Input: part model. Units: mm. Frame: model coordinates. A direction names the side the tool comes from. Give positions to 0.01 mm unless a question says otherwise; leave off trailing zeros. Write each loop counter-clockwise with the first axis right and the second up, starting at its lowest first coordinate (ties: lowest second). Pieces come first, ordered by that corner, then holes. Notation, with made-up numbers: (9, 34) - (40, 34) arc R34 cw to (40, 64) - close; hole circle Ø5 at (-37, -32.5). An arc over 180 degrees is marked (long way). Answer as a JSON object with one key per item and string values. Group by question number.
from build123d import *

# Parameters (mm, degrees)
SKETCH1_R                  = 2.430870735
SKETCH1_R_2                = 2.36295848
BASE_FLANGE1_DEPTH         = 1.0922
SKETCHED_START             = 12.060869776
SKETCHED_BEND3_OUTLINE_W   = 11.2522
SKETCHED_BEND3_OUTLINE_H   = 1.0922
SKETCHED_BEND3_DEPTH       = 16.450630224
SKETCHED_START_2           = 10.968669776
SKETCHED_BEND3_2_OUTLINE_R = 2.36295848
SKETCHED_BEND3_2_DEPTH     = 0.899042144
SKETCHED_START_3           = 10.232069776
SKETCHED_BEND3_3_OUTLINE_R = 2.36295848
SKETCHED_BEND3_3_DEPTH     = 1.8288
SKETCHED_START_4           = -5.6261
SKETCHED_BEND3_4_DEPTH     = 11.2522


with BuildPart() as part:
    # Base-Flange1: sheet metal written as solids
    # Sketch1 → Base-Flange1 (new body)
    with BuildSketch(Plane.XY):
        Polygon((-5.6261, 28.5115), (5.6261, 28.5115), (5.6261, 16.8275), (3.1242, 15.8115), (3.1242, 6.1595), (5.6261, 5.1435), (5.6261, -6.5405), (-5.6261, -6.5405), (-5.6261, 5.1435), (-3.1242, 6.1595), (-3.1242, 15.8115), (-5.6261, 16.8275), align=None)
        Circle(SKETCH1_R, mode=Mode.SUBTRACT)
        with Locations((0, 21.971)):
            Circle(SKETCH1_R_2, mode=Mode.SUBTRACT)
    extrude(amount=-BASE_FLANGE1_DEPTH)

    # Sketched Bend3: read off the stored shape, not the designer's step
    # Sketched Bend3 outline → Sketched Bend3 (cut)
    with BuildSketch(Plane(origin=(0, 0, 0), x_dir=(1, 0, 0), z_dir=(0, 1, 0)).offset(SKETCHED_START)):
        with Locations((0, 0.5461)):
            Rectangle(SKETCHED_BEND3_OUTLINE_W, SKETCHED_BEND3_OUTLINE_H)
    extrude(amount=SKETCHED_BEND3_DEPTH, mode=Mode.SUBTRACT)

    # Sketched Bend3 2 outline → Sketched Bend3 2 (add)
    with BuildSketch(Plane(origin=(0, 0, 0), x_dir=(1, 0, 0), z_dir=(0, 1, 0)).offset(SKETCHED_START_2)):
        Polygon((5.6261, 18.093369776), (-5.6261, 18.093369776), (-5.6261, 6.409369776), (-3.1242, 5.393369776), (-3.1242, 1.0922), (3.1242, 1.0922), (3.1242, 5.393369776), (5.6261, 6.409369776), align=None)
        with Locations((0, 11.552869776)):
            Circle(SKETCHED_BEND3_2_OUTLINE_R, mode=Mode.SUBTRACT)
    extrude(amount=SKETCHED_BEND3_2_DEPTH)

    # Sketched Bend3 3 outline → Sketched Bend3 3 (add)
    with BuildSketch(Plane(origin=(0, 0, 0), x_dir=(1, 0, 0), z_dir=(0, 1, 0)).offset(SKETCHED_START_3)):
        Polygon((5.6261, 18.093369776), (-5.6261, 18.093369776), (-5.6261, 6.409369776), (-3.1242, 5.393369776), (-3.1242, 1.0922), (3.1242, 1.0922), (3.1242, 5.393369776), (5.6261, 6.409369776), align=None)
        with Locations((0, 11.552869776)):
            Circle(SKETCHED_BEND3_3_OUTLINE_R, mode=Mode.SUBTRACT)
    extrude(amount=SKETCHED_BEND3_3_DEPTH)

    # Sketched Bend3 4 outline → Sketched Bend3 4 (cut)
    with BuildSketch(Plane.YZ.offset(SKETCHED_START_4)):
        with BuildLine():
            ThreePointArc((10.232069776, 0), (11.525226657, -0.535643119), (12.060869776, -1.8288))
            Line((12.060869776, -1.8288), (12.060869776, 0))
            Line((12.060869776, 0), (10.232069776, 0))
        make_face()
        with BuildLine():
            Line((10.968669776, -18.093369776), (10.968669776, -1.8288))
            ThreePointArc((10.968669776, -1.8288), (10.752924631, -1.307945145), (10.232069776, -1.0922))
            Line((10.232069776, -1.0922), (10.232069776, -18.093369776))
            Line((10.232069776, -18.093369776), (10.968669776, -18.093369776))
        make_face()
    extrude(amount=SKETCHED_BEND3_4_DEPTH, mode=Mode.SUBTRACT)


solid = part.part
1) Cut plane A-A on x = 0. Return the cut outline in (y, z), and give its area (3 significant figures).
2) Cut plane C-C on x = 1.75. Return the cut outline in (y, z).
3) Cut plane D-D on z = -8.5. Return the cut outline in (x, y).
4) Reachability of faces 5 (the face through (3.124, 9.7, -0.9)), 6 (the face through (2.32, 0.73, -0.54)), 7 (the face through (0, 10.969, -8)), 8 (the face through (-3.124, 9.7, -0.9)) from +Z, -Z, +X, -X, +Y, -Y: full face, straight path, thin tool, end or side. Return the list, or none.
5) Pin query (flat end, axial travel): P1, Ø4.5, axis at y = 10, z = -2, coming from the -X side; P2, Ø3.5, axis at x = -1, z = -12.5, coming from the -Y side; P3, Ø1.6, axis at y = 10.5, z = -2, coming from the +X side. Return the tip coordinate at first contact, or that it passes through.
6) Line query: line 1 along Y through (x, z) = (-4.5, -12.5); line 2 along Y through (x, z) = (0, -0.75); line 3 along Z through (x, y) = (0, 11.8). Output: solid intervals per line, ascending. Write a range as from..to.
7) Cut plane B-B on y = 0. Return the cut outline in (x, z), and give its area (3 significant figures).
8) Mould query, pull axis X, two halves, no side actions, for faces 1 (the face through (0, 12.061, -8)), 2 (the face through (1.09, 11.507, -9.457)), 3 (the face through (-5.626, -0.8, -0.5)), 4 (the face through (5.626, 11.5, -12.2)). Classes: +X half, -X half, draft (parallel to the pull), parting line (faces both ways), or undercut.
Filled in:
{
 "1": {"outline": "(-6.54, -1.09) - (-2.43, -1.09) - (-2.43, 0) - (-6.54, 0) - close; (2.43, -1.09) - (10.23, -1.09) arc R0.74 cw to (10.97, -1.83) - (10.97, -9.19) - (12.06, -9.19) - (12.06, -1.83) arc R1.83 ccw to (10.23, 0) - (2.43, 0) - close; (10.97, -18.09) - (12.06, -18.09) - (12.06, -13.92) - (10.97, -13.92) - close", "area": "27.8 mm²"},
 "2": {"outline": "(-6.54, -1.09) - (-1.69, -1.09) - (-1.69, 0) - (-6.54, 0) - close; (1.69, -1.09) - (10.23, -1.09) arc R0.74 cw to (10.97, -1.83) - (10.97, -9.97) - (12.06, -9.97) - (12.06, -1.83) arc R1.83 ccw to (10.23, 0) - (1.69, 0) - close; (10.97, -18.09) - (12.06, -18.09) - (12.06, -13.14) - (10.97, -13.14) - close"},
 "3": {"outline": "(-5.63, 10.97) - (5.63, 10.97) - (5.63, 12.06) - (-5.63, 12.06) - close"},
 "4": {"face 5": "+Z, +X, +Y", "face 6": "+Z, -Z", "face 7": "-Z, +X, -X, -Y", "face 8": "+Z, -X, +Y"},
 "5": {"P1": "stops at x = -3.12", "P2": "stops at y = 10.97", "P3": "stops at x = 3.12"},
 "6": {"line 1": "y = 10.97..12.06", "line 2": "y = -6.54..-2.43, 2.43..11.71", "line 3": "z = -18.09..-13.92, -9.19..-0.89"},
 "7": {"outline": "(-5.63, -1.09) - (-2.43, -1.09) - (-2.43, 0) - (-5.63, 0) - close; (2.43, -1.09) - (5.63, -1.09) - (5.63, 0) - (2.43, 0) - close", "area": "6.98 mm²"},
 "8": {"face 1": "draft", "face 2": "undercut", "face 3": "-X half", "face 4": "+X half"}
}
